Work out the finished part from the listing and answer in its coordinate system (mm). A direction names the side the tool comes from. Give positions to 0.01 mm unless a question says otherwise; leave off trailing zeros. Loops run counter-clockwise (first coordinate to the right, second up) from the corner with the lowest first, then second, coordinate; pieces in that order, holes last. Notation, with made-up numbers: (64.5, 32) - (116.5, 32) arc R28 ccw to (116.5, 60) - close; hole circle Ø6 at (-32.75, -39). An arc over 180 degrees is marked (long way). One line per question, with ' | ' between items.
from build123d import *

# Parameters (mm, degrees)
SKETCH2_W           = 42.3
SKETCH2_H           = 42.3
SKETCH2_R           = 1.7
SKETCH2_R_2         = 11.5
BOSS_EXTRUDE1_DEPTH = 4
SKETCH10_W          = 100
SKETCH10_H          = 150
BOSS_EXTRUDE3_DEPTH = 4


with BuildPart() as part:
    # Sketch2 → Boss-Extrude1 (new body)
    with BuildSketch(Plane(origin=(0, 0, 0), x_dir=(1, 0, 0), z_dir=(0, 1, 0))):
        Rectangle(SKETCH2_W, SKETCH2_H)
        with Locations(Location((-15.5, 15.5, 0), (0, 0, 270))):
            Circle(SKETCH2_R, mode=Mode.SUBTRACT)
        with Locations(Location((15.5, 15.5, 0), (0, 0, 270))):
            Circle(SKETCH2_R, mode=Mode.SUBTRACT)
        with Locations(Location((15.5, -15.5, 0), (0, 0, 270))):
            Circle(SKETCH2_R, mode=Mode.SUBTRACT)
        with Locations(Location((-15.5, -15.5, 0), (0, 0, 270))):
            Circle(SKETCH2_R, mode=Mode.SUBTRACT)
        with Locations(Location((0, 0, 0), (0, 0, 270))):
            Circle(SKETCH2_R_2, mode=Mode.SUBTRACT)
    boss_extrude1 = extrude(amount=BOSS_EXTRUDE1_DEPTH)

    # Sketch10 → Boss-Extrude3 (add)
    with BuildSketch(Plane(origin=(21.15, 4, 21.15), x_dir=(0, 0, -1), z_dir=(1, 0, 0))):
        with Locations((22.755859724, -75)):
            Rectangle(SKETCH10_W, SKETCH10_H)
    extrude(amount=BOSS_EXTRUDE3_DEPTH)

    # Mirror1: Boss-Extrude1 across plane
    add(boss_extrude1.mirror(Plane(origin=(0, -71, 0), x_dir=(0, 0, 1), z_dir=(0, -1, 0))))


solid = part.part
1. Find section B-B on x = 0. Write down the section's boundary in (y, z).
Evaluation:
outline: (-146, -21.15) - (-142, -21.15) - (-142, -11.5) - (-146, -11.5) - close; (-146, 11.5) - (-142, 11.5) - (-142, 21.15) - (-146, 21.15) - close; (0, -21.15) - (4, -21.15) - (4, -11.5) - (0, -11.5) - close; (0, 11.5) - (4, 11.5) - (4, 21.15) - (0, 21.15) - close
2. Find section A-A on z = 15.5. Write down the section's boundary in (x, y), then the cut area to 3 significant figures.
Evaluation:
outline: (-21.15, -146) - (-17.2, -146) - (-17.2, -142) - (-21.15, -142) - close; (-21.15, 0) - (-17.2, 0) - (-17.2, 4) - (-21.15, 4) - close; (-13.8, -146) - (13.8, -146) - (13.8, -142) - (-13.8, -142) - close; (-13.8, 0) - (13.8, 0) - (13.8, 4) - (-13.8, 4) - close; (17.2, -146) - (25.15, -146) - (25.15, 4) - (17.2, 4) - (17.2, 0) - (21.15, 0) - (21.15, -142) - (17.2, -142) - close | area: 884 mm2
3. Flat-ended cylindrical pins translate along their axes: pin 1 (6 mm diameter, centred on y = -65, z = -21, fed in from -X); pin 2 (2 mm diameter, centred on x = -7, y = -144, fed in from -Z); pin 3 (4.5 mm diameter, centred on x = -8.5, y = -144.5, fed in from +Z). Find the tip coordinate at first contact, or state that the pin passes through.
Evaluation:
pin 1: x = 21.15 | pin 2: z = -21.15 | pin 3: z = 21.15
4. Consider L1, parallel to X at y = 1.7, z = -15.5; L2, parallel to Y at x = 17, z = -7; L3, parallel to X at y = 1, z = 15. Determine where each line is inside the solid, lowest interval first.
Evaluation:
L1: -21.15 to -17.2, -13.8 to 13.8, 17.2 to 25.15 | L2: -146 to -142, 0 to 4 | L3: -21.15 to -17.12, -13.88 to 13.88, 17.12 to 25.15
5. Determine the mould class of faces 5 (the flat face through (-21.15, 2, 0)), 6 (the cylindrical face through (-16.15, -143.97, 17.07)), 7 (the flat face through (25.15, -70, -1)), 8 (the flat face through (23, -72, -51.606)) for opening direction X: +X half, -X half, draft (parallel to the pull), parting line (faces both ways), or undercut.
Evaluation:
face 5: -X half | face 6: undercut | face 7: +X half | face 8: draft
6. Find section C-C on z = 0. Write down the section's boundary in (x, y), then the cut area to 3 significant figures.
Evaluation:
outline: (-21.15, -146) - (-11.5, -146) - (-11.5, -142) - (-21.15, -142) - close; (-21.15, 0) - (-11.5, 0) - (-11.5, 4) - (-21.15, 4) - close; (11.5, -146) - (25.15, -146) - (25.15, 4) - (11.5, 4) - (11.5, 0) - (21.15, 0) - (21.15, -142) - (11.5, -142) - close | area: 754 mm2
7. Which of the six approach directions +Z, -Z, +X, -X, +Y, -Y give full straight-line access (tool end or side, diameter ignored) to faces 1 (the flat face through (0, 2, 21.15)), 2 (the flat face through (9, 0, 9)), 3 (the cylindrical face through (-14.99, 1.97, -13.88)), 4 (the flat face through (0, 2, -21.15))?
Evaluation:
face 1: +Z, -X, +Y, -Y | face 2: +Z, -Z, -X | face 3: +Y, -Y | face 4: -Z, -X, +Y, -Y
8. Find section D-D on x = -15.5. Write down the section's boundary in (y, z), then the cut area to 3 significant figures.
Evaluation:
outline: (-146, -21.15) - (-142, -21.15) - (-142, -17.2) - (-146, -17.2) - close; (-146, -13.8) - (-142, -13.8) - (-142, 13.8) - (-146, 13.8) - close; (-146, 17.2) - (-142, 17.2) - (-142, 21.15) - (-146, 21.15) - close; (0, -21.15) - (4, -21.15) - (4, -17.2) - (0, -17.2) - close; (0, -13.8) - (4, -13.8) - (4, 13.8) - (0, 13.8) - close; (0, 17.2) - (4, 17.2) - (4, 21.15) - (0, 21.15) - close | area: 284 mm2
